Answer from the drawing. Dimensions are ordinates in mm from the lowest x, y and z of the part. A direction names the side the tool comes from. Coordinates: 2 decimals unless noted, no trailing zeros. Loops run counter-clockwise (first coordinate to the right, second up) from the corner with the lowest first, then second, coordinate; pieces in that order, holes last. Notation, with made-up numbers: M 63,45 L 100,45 A27 cw 100,70 Z; hole C 82,-34.75 d2. An arc over 180 degrees is marked long. One line per item, written item: value. Start each with the question number.
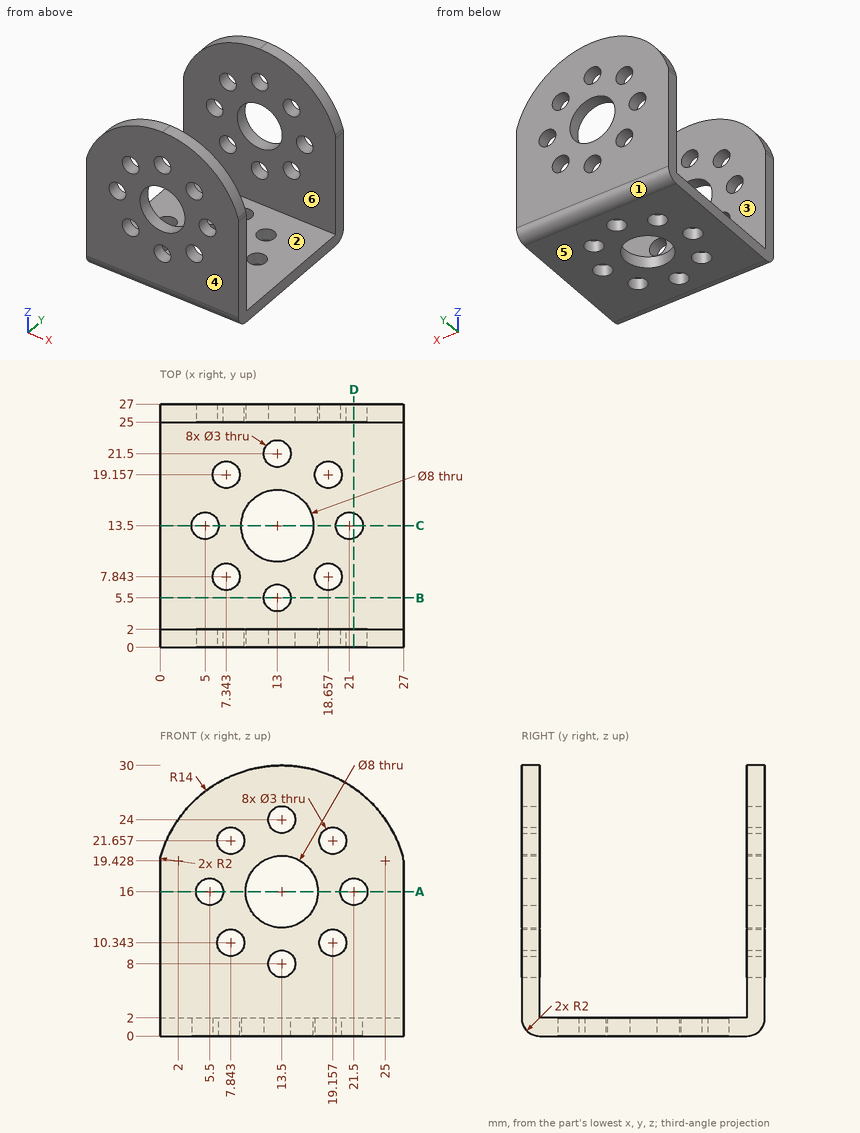
1) For a pull along Y with two mould halves and no side action, classify the marked faces 3, 4, 5 and 6 as released by +Y, released by -Y, zero draft, split by the parting line, or undercut.
2) Section D-D (x = 21.5) is taken. Determine the outline of the cut face in (y, z), then the cut area to 3 significant figures.
3) A tool of negligible diameter and unlimited length cuts with its end or side. For the marked faces 1 and 2, from which of +Z, -Z, +X, -X, +Y, -Y can it reach the whole face along a straight path? Write none if from no direction.
4) Section C-C (y = 13.5) is taken. Determine the outline of the cut face in (x, z).
5) Flat-ended cylindrical pins translate along their axes: pin 1 (4 mm diameter, centred on y = 18, z = 5, fed in from -X); pin 2 (13 mm diameter, centred on x = 13, y = 13.5, fed in from +Z); pin 3 (10 mm diameter, centred on x = 4, y = 6, fed in from +Z). Find the tip coordinate at first contact, or state that the pin passes through.
6) Consider line 1 along X through (y, z) = (13.5, 1.1); line 2 along Y through (x, z) = (3, 7); line 3 along Z through (x, y) = (7.75, 25.75) (1 decimal). Determine where each line is inside the solid, lowest interval first.
7) Section B-B (y = 5.5) is taken. Determine the outline of the cut face in (x, z), then the cut area to 3 significant figures.
8) Section A-A (z = 16) is taken. Count the separate pieces of the cut face and the enclosed holes in it, then the cut area to 3 significant figures.
Results found:
1. face 3: undercut
1. face 4: released by -Y
1. face 5: zero draft
1. face 6: undercut
2. outline: M 0,2 A2 ccw 2,0 L 12.09,0 L 12.09,2 L 2,2 L 2,14.5 L 0,14.5 Z; M 0,17.5 L 2,17.5 L 2,27.49 L 0,27.49 Z; M 14.91,0 L 25,0 A2 ccw 27,2 L 27,14.5 L 25,14.5 L 25,2 L 14.91,2 Z; M 25,17.5 L 27,17.5 L 27,27.49 L 25,27.49 Z
2. area: 137 mm²
3. face 1: -Z, +X, -X, +Y
3. face 2: +Z, +X, -X
4. outline: M 0,0 L 3.5,0 L 3.5,2 L 0,2 Z; M 6.5,0 L 9,0 L 9,2 L 6.5,2 Z; M 17,0 L 19.5,0 L 19.5,2 L 17,2 Z; M 22.5,0 L 27,0 L 27,2 L 22.5,2 Z
5. pin 1: passes through
5. pin 2: stops at z = 2
5. pin 3: stops at z = 28.4
6. line 1: x = 0 to 3.5, 6.5 to 9, 17 to 19.5, 22.5 to 27
6. line 2: y = 0 to 2, 25 to 27
6. line 3: z = 0.1 to 8.8, 11.8 to 20.2, 23.2 to 28.8
7. outline: M 0,0 L 11.5,0 L 11.5,2 L 0,2 Z; M 14.5,0 L 27,0 L 27,2 L 14.5,2 Z
7. area: 48.0 mm²
8. separate pieces: 8
8. enclosed holes: 0
8. area: 52.0 mm²
